Geometry: final body of the model. Coordinates: model frame, mm. Face numbers are marked on the shaded views. A direction names the side the tool comes from. Coordinates: 2 decimals unless noted, no trailing zeros. Write each loop counter-clockwise with the first axis right and the second up, starting at its lowest first coordinate (ties: lowest second). Pieces come first, ordered by that corner, then holes. Notation, with made-up numbers: (45.5, 54.5) - (97.5, 54.5) arc R26 ccw to (97.5, 72.5) - close; hole circle Ø9 at (87.25, -13.75). An arc over 180 degrees is marked (long way). Put each result on its own line as item: value.
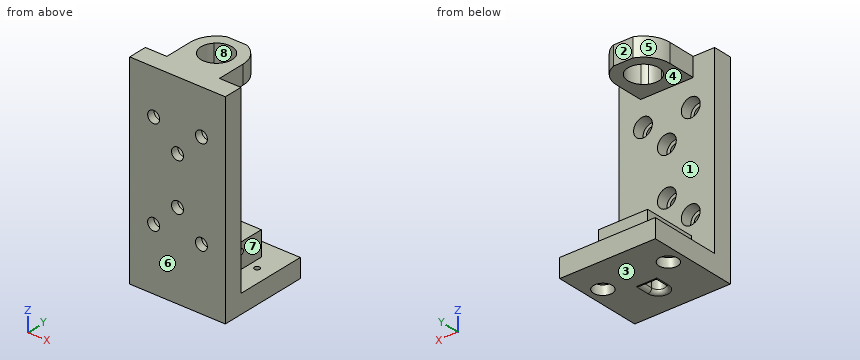
Autodesk Inventor part; units mm, degrees
ref_plane "Work Plane1" through (25.4, 10, 10) normal (1, 0, 0) x (0, 0, -1)
ref_plane "YZ Plane" through (0, 0, 0) normal (1, 0, 0) x (0, 1, 0)
ref_plane "XZ Plane" through (0, 0, 0) normal (0, 1, 0) x (-1, 0, 0)
sketch "Sketch1" plane through (0, 0, 0) normal (0, 0, 1) x (1, 0, 0)
  line L0 (0, 0) -> (0, 4)
  line L1 (0, 4) -> (0, 10)
  line L2 (0, 10) -> (0, 38)
  line L3 (0, 38) -> (0, 48)
  line L4 (0, 0) -> (50.8, 0)
  line L5 (50.8, 0) -> (50.8, 48)
  line L6 (50.8, 48) -> (0, 48)
  dimension "d1" = 4
  dimension "d2" = 6
  dimension "d3" = 28
  dimension "d4" = 10
  dimension "d5" = 50.8
extrude "Extrusion1" add sketch "Sketch1" along normal blind 10
sketch "Sketch2" plane through (0, 0, 10) normal (0, 0, 1) x (1, 0, 0)
  line L0 (50.8, 48) -> (0, 48)
  line L1 (0, 48) -> (0, 0)
  line L2 (0, 0) -> (50.8, 0)
  line L3 (50.8, 0) -> (50.8, 48)
  line L4 (0, 0) -> (50.8, 0)
  line L5 (50.8, 0) -> (50.8, 10)
  line L6 (50.8, 10) -> (0, 10)
  line L7 (0, 10) -> (0, 0)
  point P0 (0, 10)
  dimension "d8" = 10
extrude "Extrusion2" add sketch "Sketch2" along normal blind 87.5 contours L3 L2 L1 L6
sketch "Sketch3" plane through (0, 0, 10) normal (0, 0, 1) x (1, 0, 0)
  line L0 (0, 10) -> (50.8, 10)
  line L1 (50.8, 10) -> (50.8, 48)
  line L2 (50.8, 48) -> (0, 48)
  line L3 (0, 48) -> (0, 10)
  line L4 (12.4, 12) -> (38.4, 12)
  line L5 (38.4, 12) -> (38.4, 38)
  line L6 (38.4, 38) -> (12.4, 38)
  line L7 (12.4, 38) -> (12.4, 12)
  line L8 (50.8, 10) -> (0, 10)
  line L9 (38.4, 10) -> (12.4, 10)
  line L10 (12.4, 12) -> (38.4, 12)
  line L11 (38.4, 12) -> (38.4, 10)
  line L12 (38.4, 10) -> (12.4, 10)
  line L13 (12.4, 10) -> (12.4, 12)
  arc A0 (28.9, 20.1266) -> (21.9, 20.1266) centre (25.4, 25) ccw
  line L14 (19.4, 30.6624) -> (19.4, 19.3376)
  line L15 (31.4, 30.6624) -> (31.4, 19.3376)
  line L16 (23.3844, 17) -> (27.4156, 17)
  arc A1 (19.4, 19.3376) -> (23.3844, 17) centre (25.4, 25) ccw
  arc A2 (27.4156, 17) -> (31.4, 19.3376) centre (25.4, 25) ccw
  arc A3 (21.9, 18) -> (28.9, 18) centre (25.4, 18) ccw
  line L17 (21.9, 18) -> (28.9, 18)
  line L18 (28.9, 18) -> (28.9, 20.1266)
  line L19 (21.9, 20.1266) -> (21.9, 18)
  circle A4 centre (25.4, 25) radius 8.25
  point P0 (0, 0)
  point P1 (25.4, 10)
  point P2 (25.4, 12)
  point P3 (38.4, 25)
  point P4 (12.4, 25)
  point P5 (25.4, 38)
  point P6 (19.4, 25)
  point P7 (28.866, 17.5134)
  point P8 (21.934, 17.5134)
  dimension "d12" = 0
  dimension "d13" = 26
  dimension "d14" = 26
  dimension "d19" = 10
  dimension "d22" = 0
  dimension "d23" = 0
  dimension "d25" = 12
  dimension "d26" = 0
  dimension "d27" = 0
  dimension "d28" = 7
  dimension "d29" = 0
  dimension "d31" = 7
  dimension "d32" = 16.5
extrude "Extrusion3" add sketch "Sketch3" along normal blind 13 contours L13 L4 L11 L0 | L7 L6 L5 L4 | L15 A4 | L14 A4
ref_plane "Work Plane1" through (25.4, 10, 10) normal (1, 0, 0) x (0, 0, -1)
sketch "Sketch4" plane through (25.4, 10, 10) normal (1, 0, 0) x (0, 0, -1)
  line L0 (0, 20.6624) -> (0, 9.3376)
  line L1 (0, 20.6624) -> (-13, 20.6624)
  line L2 (-13, 9.3376) -> (-13, 20.6624)
  line L3 (0, 9.3376) -> (-13, 9.3376)
  circle A0 centre (-8.25, 15) radius 1.5
  point P0 (10, -10)
  point P1 (-13, 15)
  dimension "d34" = 0
  dimension "d35" = 8.25
  dimension "d36" = 3
extrude "Extrusion4" cut sketch "Sketch4" along normal mid plane 26 contours A0
sketch "Sketch5" plane through (0, 10, 97.5) normal (0, 1, 0) x (1, 0, 0)
  line L0 (12.4, 74.5) -> (12.4, 87.5)
  line L1 (0, 87.5) -> (12.4, 87.5)
  line L2 (0, 87.5) -> (0, 0)
  line L3 (50.8, 0) -> (0, 0)
  line L4 (50.8, 87.5) -> (50.8, 0)
  line L5 (38.4, 87.5) -> (50.8, 87.5)
  line L6 (38.4, 87.5) -> (38.4, 74.5)
  line L7 (38.4, 74.5) -> (12.4, 74.5)
  circle A0 centre (25.4, 51.8) radius 3.175
  line L8 (50.8, 87.5) -> (0, 87.5)
  circle A1 centre (12.7, 64.5) radius 3.175
  circle A2 centre (38.1, 64.5) radius 3.175
  line L9 (-10.8452, 39.1) -> (75.4395, 39.1)
  circle A3 centre (25.4, 26.4) radius 3.175
  circle A4 centre (12.7, 13.7) radius 3.175
  circle A5 centre (38.1, 13.7) radius 3.175
  point P0 (0, 97.5)
  point P1 (25.4, 0)
  dimension "d39" = 35.7
  dimension "d40" = 0
  dimension "d41" = 6.35
  dimension "d42" = 12.7
  dimension "d43" = 12.7
  dimension "d44" = 12.7
  dimension "d45" = 12.7
  dimension "d46" = 12.7
  dimension "d73" = 6.35
  dimension "d74" = 6.35
extrude "Extrusion5" cut sketch "Sketch5" against normal blind 26 contours A0 | A1 | A2 | A3 | A4 | A5
sketch "Sketch6" plane through (0, 0, 0) normal (0, 0, -1) x (-1, 0, 0)
  line L0 (-12.4, 10) -> (-12.4, 38)
  line L1 (-12.4, 38) -> (-38.4, 38)
  line L2 (-38.4, 38) -> (-38.4, 10)
  line L3 (-38.4, 10) -> (-50.8, 10)
  line L4 (-50.8, 10) -> (-50.8, 48)
  line L5 (-50.8, 48) -> (0, 48)
  line L6 (0, 48) -> (0, 10)
  line L7 (0, 10) -> (-12.4, 10)
  circle A0 centre (-42.8, 30) radius 1.42
  line L8 (-25.4, -18.8015) -> (-25.4, 63.6237)
  circle A1 centre (-8, 30) radius 1.42
  point P0 (0, 0)
  point P1 (-25.4, 48)
  dimension "d49" = 0
  dimension "d50" = 8
  dimension "d51" = 8
  dimension "d52" = 2.84
extrude "Extrusion6" cut sketch "Sketch6" against normal blind 26 contours A0 | A1
sketch "Sketch7" plane through (0, 0, 97.5) normal (0, 0, 1) x (1, 0, 0)
  line L0 (0, 10) -> (0, 0)
  line L1 (0, 0) -> (50.8, 0)
  line L2 (50.8, 0) -> (50.8, 10)
  line L3 (50.8, 10) -> (0, 10)
  line L4 (12.4, 38) -> (12.4, 10)
  line L5 (38.4, 10) -> (12.4, 10)
  line L6 (38.4, 10) -> (38.4, 38)
  line L7 (38.4, 38) -> (12.4, 38)
  arc A0 (31.4, 30.6624) -> (19.4, 30.6624) centre (25.4, 25) ccw
  line L8 (31.4, 30.6624) -> (31.4, 19.3376)
  arc A1 (28.866, 17.5134) -> (31.4, 19.3376) centre (25.4, 25) ccw
  arc A2 (21.934, 17.5134) -> (28.866, 17.5134) centre (25.4, 18) ccw
  arc A3 (19.4, 19.3376) -> (21.934, 17.5134) centre (25.4, 25) ccw
  line L9 (19.4, 19.3376) -> (19.4, 30.6624)
  circle A4 centre (25.4, 25) radius 14
  circle A5 centre (25.4, 25) radius 8.25
  line L10 (11.4, 25) -> (11.4, 10)
  line L11 (39.4, 25) -> (39.4, 10)
  line L12 (0, 10) -> (50.8, 10)
  line L13 (50.8, 10) -> (50.8, 0)
  line L14 (50.8, 0) -> (0, 0)
  line L15 (0, 0) -> (0, 10)
  circle A6 centre (8, 30) radius 1.42
  circle A7 centre (42.8, 30) radius 1.42
  line L16 (12.4, 10) -> (12.4, 38)
  line L17 (12.4, 38) -> (38.4, 38)
  line L18 (38.4, 38) -> (38.4, 10)
  line L19 (38.4, 10) -> (50.8, 10)
  line L20 (50.8, 10) -> (50.8, 48)
  line L21 (50.8, 48) -> (0, 48)
  line L22 (0, 48) -> (0, 10)
  line L23 (0, 10) -> (12.4, 10)
  circle A8 centre (8, 30) radius 3
  circle A9 centre (42.8, 30) radius 3
  line L24 (12.4, 38) -> (38.4, 38)
  line L25 (38.4, 38) -> (38.4, 42.0795)
  line L26 (38.4, 42.0795) -> (12.4, 42.0795)
  line L27 (12.4, 42.0795) -> (12.4, 38)
  point P0 (30.5962, 38)
  point P1 (20.2038, 38)
  dimension "d55" = 28
  dimension "d56" = 16.5
  dimension "d57" = 6
  dimension "d58" = 6
extrude "Extrusion7" add sketch "Sketch7" along normal blind 10 contours L3 L2 L1 L0 | L10 A4 L4 L3 | L4 A4 L6 L3 | A4 L4 | L6 A4 L11 L3 | L4 A4 L7 L6 | L6 A4 | A2 A5
sketch "Sketch8" plane through (0, 10, 10) normal (0, 1, 0) x (1, 0, 0)
  circle A0 centre (38.1, -73.8) radius 3.175
  circle A1 centre (38.1, -23) radius 3.175
  circle A2 centre (25.4, -61.1) radius 3.175
  circle A3 centre (25.4, -35.7) radius 3.175
  circle A4 centre (12.7, -23) radius 3.175
  circle A5 centre (12.7, -73.8) radius 3.175
  line L0 (12.4, -13) -> (12.4, 0)
  line L1 (0, 0) -> (12.4, 0)
  line L2 (0, 0) -> (0, -97.5)
  line L3 (11.4, -97.5) -> (0, -97.5)
  line L4 (11.4, -87.5) -> (11.4, -97.5)
  line L5 (39.4, -87.5) -> (11.4, -87.5)
  line L6 (39.4, -87.5) -> (39.4, -97.5)
  line L7 (50.8, -97.5) -> (39.4, -97.5)
  line L8 (50.8, 0) -> (50.8, -97.5)
  line L9 (38.4, 0) -> (50.8, 0)
  line L10 (38.4, 0) -> (38.4, -13)
  line L11 (38.4, -13) -> (12.4, -13)
  circle A6 centre (25.4, -35.7) radius 5
  circle A7 centre (12.7, -23) radius 5
  circle A8 centre (38.1, -23) radius 5
  circle A9 centre (25.4, -61.1) radius 5
  circle A10 centre (12.7, -73.8) radius 3.175
  circle A11 centre (12.7, -73.8) radius 5
  circle A12 centre (38.1, -73.8) radius 5
  point P0 (0, 10)
  dimension "d61" = 10
  dimension "d62" = 10
  dimension "d63" = 10
  dimension "d64" = 10
  dimension "d65" = 10
  dimension "d66" = 10
extrude "Extrusion8" cut sketch "Sketch8" against normal blind 6 contours A2 | A6 | A7 | A8 | A9 | A11 | A12
sketch "Sketch9" plane through (0, 0, 0) normal (0, 0, -1) x (-1, 0, 0)
  circle A0 centre (-8, 30) radius 1.42
  circle A1 centre (-42.8, 30) radius 1.42
  line L0 (-50.8, 48) -> (0, 48)
  line L1 (-50.8, 0) -> (-50.8, 48)
  line L2 (0, 0) -> (-50.8, 0)
  line L3 (0, 48) -> (0, 0)
  circle A2 centre (-42.8, 30) radius 5
  circle A3 centre (-8, 30) radius 5
  dimension "d69" = 10
  dimension "d70" = 10
extrude "Extrusion9" cut sketch "Sketch9" against normal blind 5 contours A1 | A2 | A3
sketch "Sketch10" plane through (0, 0, 23) normal (0, 0, 1) x (1, 0, 0)
  line L0 (12.4, 38) -> (12.4, 10)
  line L1 (38.4, 10) -> (12.4, 10)
  line L2 (38.4, 10) -> (38.4, 38)
  line L3 (38.4, 38) -> (12.4, 38)
  arc A0 (31.4, 30.6624) -> (19.4, 30.6624) centre (25.4, 25) ccw
  line L4 (31.4, 30.6624) -> (31.4, 19.3376)
  arc A1 (28.866, 17.5134) -> (31.4, 19.3376) centre (25.4, 25) ccw
  arc A2 (21.934, 17.5134) -> (28.866, 17.5134) centre (25.4, 18) ccw
  arc A3 (19.4, 19.3376) -> (21.934, 17.5134) centre (25.4, 25) ccw
  line L5 (19.4, 19.3376) -> (19.4, 30.6624)
  circle A4 centre (25.4, 15.5) radius 3.5
  line L6 (21.9, 15.5) -> (28.9, 15.5)
  line L7 (28.9, 15.5) -> (28.9, 21)
  line L8 (28.9, 21) -> (21.9, 21)
  line L9 (21.9, 21) -> (21.9, 15.5)
  point P0 (0, 0)
  dimension "d75" = 7
  dimension "d76" = 5.5
  dimension "d77" = 0
  dimension "d78" = 7
  dimension "d79" = 5.5
extrude "Extrusion10" cut sketch "Sketch10" against normal through all contours L7 A4 A2 A1 | A1 A2 A4 A3 L9 L8 L7 | A3 A2 A4 L9 | L6 A2 A4 | A4 L6 A2 | A4 A2 L6 | A2 L6 A4 | A2 L6
fillet "Fillet1" radius 2 7 edges at (25.4, 21, 10) (21.9, 19.2646, 10) (28.9, 19.2646, 10) (28.9, 18.25, 0) (21.9, 18.25, 0) (25.4, 12, 0) (25.4, 21, 0)
equation "\"d4\" = Thick_Wall"
equation "\"d5\" = Platform_Width"
equation "\"d6\" = Thick_Wall"
equation "\"d8\" = d1 + d2"
equation "\"d19\" = Thick_Wall"
equation "\"d41\" = Tabletop_Hole_Diameter"
equation "\"d42\" = d43"
equation "\"d43\" = 0.5 * Tabletop_Hole_Spacing"
equation "\"d44\" = d43"
equation "\"d45\" = d43"
equation "\"d46\" = d43"
equation "\"d73\" = d41"
equation "\"d74\" = d41"
equation "\"d57\" = Guide_Rod_Diameter"
equation "\"d58\" = Guide_Rod_Diameter"
equation "\"d59\" = Thick_Wall"
equation "\"d62\" = d61"
equation "\"d63\" = d61"
equation "\"d64\" = d61"
equation "\"d65\" = d61"
equation "\"d66\" = d61"
equation "\"d67\" = d2"
equation "\"d71\" = 0.5 * Thick_Wall"
equation "\"d78\" = d75"
equation "\"Platform_Width\" = 50.8"
equation "\"Platform_Length\" = 245"
equation "\"Guide_Hole_Offset\" = 13.51"
equation "\"Guide_Rod_Diameter\" = 6"
equation "\"Guide_Rod_Length\" = 304.8"
equation "\"Thin_Wall\" = 5"
equation "\"Thick_Wall\" = 10"
equation "\"Tabletop_Hole_Spacing\" = 25.4"
equation "\"Tabletop_Hole_Diameter\" = 6.35"
equation "\"Platform_Hole_Spacing\" = 25.4"
equation "\"Platform_Hole_Diameter\" = 6.35"
equation "\"d15\" = Thin_Wall"
equation "\"d17\" = d15"
equation "\"Actuator_Housing_W\" = 26"
equation "\"Sliding_Clearance\" = 2"
equation "\"Platform_GuideRod_OD\" = 16.5"
properties part number "Actuator Mount"
1. Section query C-C (z = 14). Return loops of the section in (x, y).
Answer below:
outline: (0, 0) - (50.8, 0) - (50.8, 10) - (38.4, 10) - (38.4, 38) - (12.4, 38) - (12.4, 10) - (0, 10) - close; hole (19.4, 19.34) arc R8.25 ccw to (21.9, 17.53) - (21.9, 15.5) arc R3.5 ccw to (28.9, 15.5) - (28.9, 17.53) arc R8.25 ccw to (31.4, 19.34) - (31.4, 30.66) arc R8.25 ccw to (19.4, 30.66) - close
2. Section query D-D (x = 25.4). Count the separate pieces of the cut face and the enclosed holes in it, then the cut area to 3 significant figures.
Answer below:
separate pieces: 5
enclosed holes: 0
area: 1,390 mm²
3. Ray query, probe 1 along Y at (x, z) = (42.8, 6.75); probe 2 along X at (y, z) = (25, 16); probe 3 along Y at (x, z) = (25, 6.5). Return the intervals inside material, ascending. Write a range as from..to.
Answer below:
probe 1: y = 0..28.58, 31.42..48
probe 2: x = 12.4..19.4, 31.4..38.4
probe 3: y = 0..12.02, 21..48
4. Section query A-A (z = 45.7). Return loops of the section in (x, y) (3 decimals).
Answer below:
outline: (0, 0) - (22.225, 0) - (22.225, 4) - (20.4, 4) - (20.4, 10) - (0, 10) - close; (28.575, 0) - (50.8, 0) - (50.8, 10) - (30.4, 10) - (30.4, 4) - (28.575, 4) - close
5. Section query B-B (z = 83.8). Return loops of the section in (x, y) (3 decimals).
Answer below:
outline: (0, 0) - (9.525, 0) - (9.525, 4) - (7.7, 4) - (7.7, 10) - (0, 10) - close; (15.875, 0) - (34.925, 0) - (34.925, 4) - (33.1, 4) - (33.1, 10) - (17.7, 10) - (17.7, 4) - (15.875, 4) - close; (41.275, 0) - (50.8, 0) - (50.8, 10) - (43.1, 10) - (43.1, 4) - (41.275, 4) - close
6. Mould query, pull axis Z, two halves, no side actions, for the marked faces 1, 2, 3 and 4. Classes: +Z half, -Z half, draft (parallel to the pull), parting line (faces both ways), or undercut.
Answer below:
face 1: undercut
face 2: draft
face 3: -Z half
face 4: undercut
7. Set-up query: the marked faces 5, 6, 7 and 8. Return all of +Z, -Z, +X, -X, +Y, -Y with unobstructed straight access to the full face (end or side cutting, diameter ignored); none if empty.
Answer below:
face 5: +Z, -X, +Y
face 6: +Z, -Z, +X, -X, -Y
face 7: +X, +Y
face 8: +Z
8. Pin query (flat end, axial travel): pin 1 Ø1.5 at (x, z) = (10, 35.5) entering from +Y; pin 2 Ø10 at (x, y) = (45, 20.5) entering from +Z; pin 3 Ø2 at (x, z) = (42, 43) entering from +Y; pin 4 Ø3 at (x, z) = (24.5, 70.5) entering from +Y. Return the tip coordinate at first contact, or that it passes through.
Answer below:
pin 1: stops at y = 4
pin 2: stops at z = 10
pin 3: stops at y = 10
pin 4: passes through
